Autodesk Inventor part; units mm, degrees
ref_plane "YZ Plane" through (0, 0, 0) normal (1, 0, 0) x (0, 1, 0)
ref_plane "XZ Plane" through (0, 0, 0) normal (0, 1, 0) x (-1, 0, 0)
ref_plane "XY Plane" through (0, 0, 0) normal (0, 0, 1) x (1, 0, 0)
sketch "Sketch1" plane through (0, 0, 0) normal (1, 0, 0) x (0, 1, 0)
  line L0 (10.75, 26) -> (-6.5, 26)
  arc A0 (-6.5, 26) -> (-7, 25.5) centre (-6.5, 25.5) ccw
  line L1 (-7, 25.5) -> (-7, 7)
  arc A1 (-7, 7) -> (0, 0) centre (0, 7) ccw
  line L2 (0, 0) -> (22, 0)
  arc A2 (22, 0) -> (29, 7) centre (22, 7) ccw
  line L3 (29, 7) -> (29, 25.5)
  arc A3 (29, 25.5) -> (28.5, 26) centre (28.5, 25.5) ccw
  line L4 (28.5, 26) -> (-6.5, 26)
  circle A4 centre (0, 7) radius 2.25
  circle A5 centre (22, 7) radius 2.25
  point P0 (0, 0)
  point P1 (-7, 7)
  point P2 (0, 0)
extrude "Extrusion1" add sketch "Sketch1" along normal blind 12.192
Input: part model. Units: mm. Frame: model coordinates. Give positions to 0.01 mm unless a question says otherwise; leave off trailing zeros. Write each loop counter-clockwise with the first axis right and the second up, starting at its lowest first coordinate (ties: lowest second). Pieces come first, ordered by that corner, then holes.
Q1. Pull-direction query (Y, two-part tool) for faces 1 (the face through (6, 29, 16)), 2 (the face through (0, 11, 13)), 3 (the face through (6.01, -0.29, 4.77)); classes: pulls with the +Y half, pulls with the -Y half, needs draft (parallel to the pull), parting line crosses it, or undercut.
Q2. First-contact query: P1, Ø3.5, axis at y = 22, z = 7, coming from the -X side. Flat tip, straight axial feed; report the tip coordinate or a pass-through.
Q3. Section A-A, the plane x = 7.5. Output: boundary loops of the cut face in (y, z), plus the area to 3 significant figures.
Q4. Material intervals for probe 1 along Z at (x, y) = (8.75, 22); probe 2 along Y at (x, z) = (1.5, 8); probe 3 along Y at (x, z) = (8, 2.25), sorted ascending.
Filled in:
1. face 1: pulls with the +Y half
1. face 2: needs draft
1. face 3: undercut
2. P1: passes through
3. outline: (-7, 7) arc R7 ccw to (0, 0) - (22, 0) arc R7 ccw to (29, 7) - (29, 25.5) arc R0.5 ccw to (28.5, 26) - (-6.5, 26) arc R0.5 ccw to (-7, 25.5) - close; hole circle Ø4.5 at (0, 7); hole circle Ø4.5 at (22, 7)
3. area: 883 mm2
4. probe 1: z = 0 to 4.75, 9.25 to 26
4. probe 2: y = -7 to -2.02, 2.02 to 19.98, 24.02 to 29
4. probe 3: y = -5.14 to 27.14
